Can you work these out from the model? Positions are in its coordinate system, mm. A direction names the side the tool comes from. Give positions to 0.01 mm unless a question says otherwise; leave off trailing zeros. Order: outer loops, then holes, each group sorted by start corner. A loop starts at its lowest first (then second) coordinate and runs counter-clockwise, first axis right, second up. Notation, with made-up numbers: (28.25, 9.5) - (55.25, 9.5) arc R17 ccw to (55.25, 24.5) - close; hole circle Ø4 at (66, -35). An arc over 180 degrees is marked (long way). Use one line per item in the form item = value. Start each with the question number.
1) We'd pull the mould along X, two halves only. Please class faces 4 (the flat face through (17.4, 10, 7.6)), 5 (the cylindrical face through (17.27, 5.07, 8.5)), 6 (the cylindrical face through (32.15, 13.01, 9.86)): released by +X, released by -X, zero draft, split by the parting line, or undercut.
2) Suppose I cut it at C-C, the plane z = 18.5. Write out the boundary of the cut face in (x, y).
3) Please list where these lines run through material, in increasing order: probe 1 along Y at (x, z) = (45, 14.25); probe 2 along Y at (x, z) = (44.5, 9); probe 3 along X at (y, z) = (4.5, 10).
4) For pin 1 (1 mm diameter, centred on x = 34, y = 53.5, fed in from +Z); pin 2 (12 mm diameter, centred on y = 63.5, z = 5.5, fed in from -X); pin 3 (10 mm diameter, centred on x = 17.5, z = 6.5, fed in from +Y); pin 4 (2.5 mm diameter, centred on x = 45, y = 20, fed in from +Z), each with a flat end and sliding along its axis, tell me the tip position at first contact or that it passes through.
5) Suppose I cut it at B-B, the plane x = 12.5. Write out the boundary of the cut face in (y, z).
6) Which directions (+Z, -Z, +X, -X, +Y, -Y) give clear straight access to the entire face, cutting with the end or side of a thin tool? Please do faces 1 (the flat face through (35, 86, 10)), 2 (the flat face through (41, 76, 20)), 3 (the cylindrical face through (43.9, 131.19, 14.02)).
7) Suppose I cut it at D-D, the plane y = 110.5. Write out the boundary of the cut face in (x, z).
8) Suppose I cut it at A-A, the plane z = 10. Write out the boundary of the cut face in (x, y), and give its area (3 significant figures).
Autodesk Inventor part; units mm, degrees
ref_plane "YZ Plane" through (0, 0, 0) normal (1, 0, 0) x (0, 1, 0)
ref_plane "XZ Plane" through (0, 0, 0) normal (0, 1, 0) x (-1, 0, 0)
ref_plane "XY Plane" through (0, 0, 0) normal (0, 0, 1) x (1, 0, 0)
sketch "Bracket Tall" plane through (0, 0, 0) normal (0, 0, 1) x (1, 0, 0)
  line L0 (0, 0) -> (30, 0)
  line L1 (25, 10) -> (0, 10)
  line L2 (0, 10) -> (0, 0)
  line L3 (30, 0) -> (55, 0)
  line L4 (55, 0) -> (55, 150)
  line L5 (55, 150) -> (35, 150)
  line L6 (35, 150) -> (35, 20)
  arc A0 (25, 10) -> (35, 20) centre (25, 20) ccw
  point P0 (35, 10)
  dimension "d0" = 35
  dimension "d2" = 20
  dimension "d3" = 150
  dimension "d4" = 10
  dimension "d10" = 10
extrude "Extrusion1" add sketch "Bracket Tall" along normal blind 20
sketch "Clearance Hole (M6-8)" plane through (0, 10, 0) normal (0, 1, 0) x (1, 0, 0)
  circle A0 centre (12.5, -10) radius 5
  line L0 (0, 0) -> (0, -20)
  line L1 (25, 0) -> (25, -20)
  dimension "d7" = 10
extrude "Extrusion2" cut sketch "Clearance Hole (M6-8)" against normal through all
sketch "Sketch4" plane through (0, 0, 20) normal (0, 0, 1) x (1, 0, 0)
  circle A0 centre (45, 20) radius 1.621
  circle A1 centre (45, 20) radius 1.621
  line L0 (45, 20) -> (45, 130)
  point P0 (0, 0)
  dimension "d34" = 110
hole "Hole2" at (45, 20, 20) at (45, 130, 20) direction (0, 0, -1) diameter 3.242 depth 11.8 tip angle 118
move faces "Move1" translate (5, 0, 0) faces at (0, 6.6667, 6.6667)
properties part number "Bracket_Tall2" material "Aluminum, Anodized Silver"
Result sheet:
q1.face_4 = zero draft
q1.face_5 = undercut
q1.face_6 = released by -X
q2.outline = (5, 0) - (55, 0) - (55, 150) - (35, 150) - (35, 20) arc R10 cw to (25, 10) - (5, 10) - close; hole circle Ø3.24 at (45, 20); hole circle Ø3.24 at (45, 130)
q3.probe_1 = 0 to 18.38, 21.62 to 128.38, 131.62 to 150
q3.probe_2 = 0 to 18.46, 21.54 to 128.46, 131.54 to 150
q3.probe_3 = 5 to 7.5, 17.5 to 55
q4.pin_1 = through
q4.pin_2 = 35
q4.pin_3 = 10
q4.pin_4 = 7.98
q5.outline = (0, 0) - (10, 0) - (10, 5) - (0, 5) - close; (0, 15) - (10, 15) - (10, 20) - (0, 20) - close
q6.face_1 = +Z, -Z, -X, +Y
q6.face_2 = +Z, +X, -X, +Y, -Y
q6.face_3 = +Z
q7.outline = (35, 0) - (55, 0) - (55, 20) - (35, 20) - close
q8.outline = (5, 0) - (7.5, 0) - (7.5, 10) - (5, 10) - close; (17.5, 0) - (55, 0) - (55, 150) - (35, 150) - (35, 20) arc R10 cw to (25, 10) - (17.5, 10) - close; hole circle Ø3.24 at (45, 20); hole circle Ø3.24 at (45, 130)
q8.area = 3,200 mm²
